```python
from build123d import *

# Parameters (mm, degrees)
SKETCH2_R                                  = 87.5
BOSS_EXTRUDE2_DEPTH                        = 2
SKETCH3_W                                  = 55
SKETCH3_H                                  = 40
CUT_EXTRUDE1_DEPTH                         = 124.759848093
CUT_EXTRUDE2_DEPTH                         = 124.759848093
SKETCH7_R                                  = 1.75
CUT_EXTRUDE3_DEPTH                         = 124.759848093
MIRROR1_AT_THE_SECOND_PLANE_COPY_1_DEPTH   = 124.759848093
MIRROR1_AT_THE_SECOND_PLANE_COPY_2_SKETC_R = 1.75
MIRROR1_AT_THE_SECOND_PLANE_COPY_2_DEPTH   = 124.759848093
SKETCH8_W                                  = 50
SKETCH8_H                                  = 15
CUT_EXTRUDE5_DEPTH                         = 124.759848093
SKETCH11_R                                 = 1.75
CUT_EXTRUDE7_DEPTH                         = 124.759848093
LPATTERN2_COUNT                            = 3
LPATTERN2_PITCH                            = 20
CIRPATTERN1_COUNT                          = 3
CIRPATTERN1_ANGLE                          = 180
CIRPATTERN1_COPY_1_SKETCH_R                = 1.75
CIRPATTERN1_COPY_1_DEPTH                   = 124.759848093
CIRPATTERN1_COPY_2_SKETCH_R                = 1.75
CIRPATTERN1_COPY_2_DEPTH                   = 124.759848093
CIRPATTERN1_COPY_3_SKETCH_R                = 1.75
CIRPATTERN1_COPY_3_DEPTH                   = 124.759848093
CIRPATTERN1_COPY_4_SKETCH_R                = 1.75
CIRPATTERN1_COPY_4_DEPTH                   = 124.759848093
SKETCH13_W                                 = 15
SKETCH13_H                                 = 50
CUT_EXTRUDE8_DEPTH                         = 124.759848093
SKETCH14_R                                 = 1.75
CUT_EXTRUDE9_DEPTH                         = 124.759848093


with BuildPart() as part:
    # Sketch2 → Boss-Extrude2 (new body)
    with BuildSketch(Plane.XY):
        Circle(SKETCH2_R)
    extrude(amount=BOSS_EXTRUDE2_DEPTH)

    # Sketch3 → Cut-Extrude1 (cut, through all)
    with BuildSketch(Plane.XY.offset(2)):
        with Locations((0, 87.5)):
            Rectangle(SKETCH3_W, SKETCH3_H)
    extrude(amount=-CUT_EXTRUDE1_DEPTH, mode=Mode.SUBTRACT)

    # Sketch6 → Cut-Extrude2 (cut, through all)
    with BuildSketch(Plane.XY.offset(2)):
        with BuildLine():
            Line((-79.237656457, 37.116624298), (-66.214900923, 26.189234933))
            Line((-66.214900923, 26.189234933), (-62.036781461, 31.168523814))
            Line((-62.036781461, 31.168523814), (-49.014025927, 20.241134449))
            Line((-49.014025927, 20.241134449), (-28.444822418, 44.754556629))
            Line((-28.444822418, 44.754556629), (-41.467577951, 55.681945993))
            Line((-41.467577951, 55.681945993), (-37.289458488, 60.661234874))
            Line((-37.289458488, 60.661234874), (-50.312214021, 71.588624238))
            ThreePointArc((-50.312214021, 71.588624238), (-67.028888773, 56.243915848), (-79.237656457, 37.116624298))
        make_face()
    cut_extrude2 = extrude(amount=-CUT_EXTRUDE2_DEPTH, mode=Mode.SUBTRACT)

    # Sketch7 → Cut-Extrude3 (cut, through all)
    with BuildSketch(Plane.XY.offset(2)):
        with Locations((-61.645137707, 14.522304568)):
            Circle(SKETCH7_R)
        with Locations((-25.006243955, 58.186837826)):
            Circle(SKETCH7_R)
    cut_extrude3 = extrude(amount=-CUT_EXTRUDE3_DEPTH, mode=Mode.SUBTRACT)

    # Mirror1: Cut-Extrude2, Cut-Extrude3 across plane
    add(cut_extrude2.mirror(Plane.ZX), mode=Mode.SUBTRACT)
    add(cut_extrude3.mirror(Plane.ZX), mode=Mode.SUBTRACT)

    # Mirror1 at the second plane: Cut-Extrude2, Cut-Extrude3 across plane
    add(cut_extrude2.mirror(Plane(origin=(0, 0, 0), x_dir=(0, 0, 1), z_dir=(1, 0, 0))), mode=Mode.SUBTRACT)
    add(cut_extrude3.mirror(Plane(origin=(0, 0, 0), x_dir=(0, 0, 1), z_dir=(1, 0, 0))), mode=Mode.SUBTRACT)

    # Mirror1 at the second plane copy 1 sketc → Mirror1 at the second plane copy 1 (cut, through all)
    with BuildSketch(Plane(origin=(0, 0, 2), x_dir=(-1, 0, 0), z_dir=(0, 0, 1))):
        with BuildLine():
            Line((-79.237656457, 37.116624298), (-66.214900923, 26.189234933))
            Line((-66.214900923, 26.189234933), (-62.036781461, 31.168523814))
            Line((-62.036781461, 31.168523814), (-49.014025927, 20.241134449))
            Line((-49.014025927, 20.241134449), (-28.444822418, 44.754556629))
            Line((-28.444822418, 44.754556629), (-41.467577951, 55.681945993))
            Line((-41.467577951, 55.681945993), (-37.289458488, 60.661234874))
            Line((-37.289458488, 60.661234874), (-50.312214021, 71.588624238))
            ThreePointArc((-50.312214021, 71.588624238), (-67.028888773, 56.243915848), (-79.237656457, 37.116624298))
        make_face()
    extrude(amount=-MIRROR1_AT_THE_SECOND_PLANE_COPY_1_DEPTH, mode=Mode.SUBTRACT)

    # Mirror1 at the second plane copy 2 sketc → Mirror1 at the second plane copy 2 (cut, through all)
    with BuildSketch(Plane(origin=(0, 0, 2), x_dir=(-1, 0, 0), z_dir=(0, 0, 1))):
        with Locations((-61.645137707, 14.522304568)):
            Circle(MIRROR1_AT_THE_SECOND_PLANE_COPY_2_SKETC_R)
        with Locations((-25.006243955, 58.186837826)):
            Circle(MIRROR1_AT_THE_SECOND_PLANE_COPY_2_SKETC_R)
    extrude(amount=-MIRROR1_AT_THE_SECOND_PLANE_COPY_2_DEPTH, mode=Mode.SUBTRACT)

    # Sketch8 → Cut-Extrude5 (cut, through all)
    with BuildSketch(Plane.XY.offset(2)):
        with Locations((-55, 0)):
            Rectangle(SKETCH8_W, SKETCH8_H)
    cut_extrude5 = extrude(amount=-CUT_EXTRUDE5_DEPTH, mode=Mode.SUBTRACT)

    # Sketch11 → Cut-Extrude7 (cut, through all)
    with BuildSketch(Plane.XY.offset(2)):
        with Locations((-35, 10.5)):
            Circle(SKETCH11_R)
        with Locations((-35, -10.5)):
            Circle(SKETCH11_R)
    cut_extrude7 = extrude(amount=-CUT_EXTRUDE7_DEPTH, mode=Mode.SUBTRACT)

    # LPattern2: Cut-Extrude7 ×3
    with Locations(*[(-i * LPATTERN2_PITCH, 0, 0) for i in range(1, LPATTERN2_COUNT)]):
        add(cut_extrude7, mode=Mode.SUBTRACT)

    # CirPattern1: Cut-Extrude5, Cut-Extrude7 ×3 about axis
    cirpattern1_axis = Axis((0, 0, 0), (0, 0, 1))
    add([cut_extrude5.rotate(cirpattern1_axis, i * CIRPATTERN1_ANGLE / (CIRPATTERN1_COUNT - 1)) for i in range(1, CIRPATTERN1_COUNT)], mode=Mode.SUBTRACT)
    add([cut_extrude7.rotate(cirpattern1_axis, i * CIRPATTERN1_ANGLE / (CIRPATTERN1_COUNT - 1)) for i in range(1, CIRPATTERN1_COUNT)], mode=Mode.SUBTRACT)

    # CirPattern1 copy 1 sketch → CirPattern1 copy 1 (cut, through all)
    with BuildSketch(Plane(origin=(0, -20, 2), x_dir=(0, 1, 0), z_dir=(0, 0, 1))):
        with Locations((-35, 10.5)):
            Circle(CIRPATTERN1_COPY_1_SKETCH_R)
        with Locations((-35, -10.5)):
            Circle(CIRPATTERN1_COPY_1_SKETCH_R)
    extrude(amount=-CIRPATTERN1_COPY_1_DEPTH, mode=Mode.SUBTRACT)

    # CirPattern1 copy 2 sketch → CirPattern1 copy 2 (cut, through all)
    with BuildSketch(Plane(origin=(20, 0, 2), x_dir=(-1, 0, 0), z_dir=(0, 0, 1))):
        with Locations((-35, 10.5)):
            Circle(CIRPATTERN1_COPY_2_SKETCH_R)
        with Locations((-35, -10.5)):
            Circle(CIRPATTERN1_COPY_2_SKETCH_R)
    extrude(amount=-CIRPATTERN1_COPY_2_DEPTH, mode=Mode.SUBTRACT)

    # CirPattern1 copy 3 sketch → CirPattern1 copy 3 (cut, through all)
    with BuildSketch(Plane(origin=(0, -40, 2), x_dir=(0, 1, 0), z_dir=(0, 0, 1))):
        with Locations((-35, 10.5)):
            Circle(CIRPATTERN1_COPY_3_SKETCH_R)
        with Locations((-35, -10.5)):
            Circle(CIRPATTERN1_COPY_3_SKETCH_R)
    extrude(amount=-CIRPATTERN1_COPY_3_DEPTH, mode=Mode.SUBTRACT)

    # CirPattern1 copy 4 sketch → CirPattern1 copy 4 (cut, through all)
    with BuildSketch(Plane(origin=(40, 0, 2), x_dir=(-1, 0, 0), z_dir=(0, 0, 1))):
        with Locations((-35, 10.5)):
            Circle(CIRPATTERN1_COPY_4_SKETCH_R)
        with Locations((-35, -10.5)):
            Circle(CIRPATTERN1_COPY_4_SKETCH_R)
    extrude(amount=-CIRPATTERN1_COPY_4_DEPTH, mode=Mode.SUBTRACT)

    # Sketch13 → Cut-Extrude8 (cut, through all)
    with BuildSketch(Plane.XY.offset(2)):
        with Locations((0, 32.5)):
            Rectangle(SKETCH13_W, SKETCH13_H)
    extrude(amount=-CUT_EXTRUDE8_DEPTH, mode=Mode.SUBTRACT)

    # Sketch14 → Cut-Extrude9 (cut, through all)
    with BuildSketch(Plane.XY.offset(2)):
        with Locations((-15, 42.5)):
            Circle(SKETCH14_R)
        with Locations((15, 42.5)):
            Circle(SKETCH14_R)
        with Locations((-15, 36.5)):
            Circle(SKETCH14_R)
        with Locations((15, 36.5)):
            Circle(SKETCH14_R)
        with Locations((-15, 30.5)):
            Circle(SKETCH14_R)
        with Locations((15, 30.5)):
            Circle(SKETCH14_R)
        with Locations((-15, 24.5)):
            Circle(SKETCH14_R)
        with Locations((15, 24.5)):
            Circle(SKETCH14_R)
        with Locations((-15, 18.5)):
            Circle(SKETCH14_R)
        with Locations((15, 18.5)):
            Circle(SKETCH14_R)
        with Locations((-15, 12.5)):
            Circle(SKETCH14_R)
        with Locations((15, 12.5)):
            Circle(SKETCH14_R)
        with Locations((-15, 6.5)):
            Circle(SKETCH14_R)
        with Locations((15, 6.5)):
            Circle(SKETCH14_R)
        with Locations((-15, 0.5)):
            Circle(SKETCH14_R)
        with Locations((15, 0.5)):
            Circle(SKETCH14_R)
    extrude(amount=-CUT_EXTRUDE9_DEPTH, mode=Mode.SUBTRACT)


solid = part.part
```
Input: part model. Units: mm. Frame: model coordinates. A direction names the side the tool comes from. Round coordinates to 2 decimals unless told otherwise and drop trailing zeros. Loops run counter-clockwise (first coordinate to the right, second up) from the corner with the lowest first, then second, coordinate; pieces in that order, holes last. Notation, with made-up numbers: (-24.75, 57) - (30.25, 57) arc R20 ccw to (30.25, 61) - close; hole circle Ø6 at (34.25, 28). An arc over 180 degrees is marked (long way). One line per item, written item: value. Start each with the question number.
(1) Ray query, line 1 (Y direction, x = -1, z = 0.9); line 2 (Y direction, x = 34.5, z = 0.8); line 3 (X direction, y = -75, z = 0.55). Return the intervals inside material, ascending. Write a range as [from, to].
(2) Section A-A, the plane x = 5. Return loops of the section in (y, z).
(3) Draft query along X for faces 1 (the cylindrical face through (87.5, -0.5, 1)), 2 (the flat face through (38.87, -32.33, 1.01)), 3 (the flat face through (-1, -1, 0)). Return one class per face: +X half, -X half, draft (parallel to the pull), parting line (faces both ways), or undercut.
(4) Section C-C, the plane z = 0.5. Count the separate pieces of the cut face and the enclosed holes in it, plus the area to 3 significant figures.
(5) Section B-B, the plane y = -5.5. Return loops of the section in (x, z), plus the area to 3 significant figures.
(6) Contact query for flat-ended pins moving along their axis: P1, Ø4, axis at x = 75, y = -10.5, coming from the +Z side; P2, Ø1, axis at x = 59, z = 1.5, coming from the -Y side; P3, Ø1, axis at y = 58, z = 1.5, coming from the +X side; P4, Ø0.6, axis at y = -3, z = 0.5, coming from the +X side. Output: stop coordinate, or through.
(7) Access query for faces 4 (the flat face through (-64.16, -28.64, 1.01)), 5 (the flat face through (-39.408, 58.137, 1.014)), 6 (the flat face through (38.87, 32.33, 1.01)), 7 (the flat face through (43.71, -66.05, 1.01)). Directions: +Z, -Z, +X, -X, +Y, -Y. A direction counts if a zero-diameter tool reaches every point of the face in a straight line with its end or side. Return the directions, or none.
Results below:
1. line 1: [-87.49, -80], [-30, 7.5], [57.5, 67.5]
1. line 2: [-80.41, -49.84], [-37.54, -12.18], [-8.82, -7.5], [7.5, 8.82], [12.18, 37.54], [49.84, 80.41]
1. line 3: [-45.07, -12.25], [-8.75, -7.5], [7.5, 8.75], [12.25, 45.07]
2. outline: (-87.36, 0) - (-80, 0) - (-80, 2) - (-87.36, 2) - close; (-30, 0) - (7.5, 0) - (7.5, 2) - (-30, 2) - close; (57.5, 0) - (67.5, 0) - (67.5, 2) - (57.5, 2) - close
3. face 1: +X half
3. face 2: undercut
3. face 3: draft
4. separate pieces: 1
4. enclosed holes: 46
4. area: 14,000 mm^2
5. outline: (-87.33, 0) - (-80, 0) - (-80, 2) - (-87.33, 2) - close; (-30, 0) - (30, 0) - (30, 2) - (-30, 2) - close; (80, 0) - (87.33, 0) - (87.33, 2) - (80, 2) - close
5. area: 149 mm^2
6. P1: z = 2
6. P2: y = -29.04
6. P3: x = 39.94
6. P4: x = 87.46
7. face 4: +Z, -Z, -Y
7. face 5: +Z, -Z, -X
7. face 6: +Z, -Z
7. face 7: +Z, -Z, +X
